Autodesk Fusion 360 part; units mm, degrees
sketch "base" plane through (0, 0, 0) normal (0, 0, 1) x (1, 0, 0)
  circle A0 centre (0, 0) radius 48
  circle A1 centre (0, 0) radius 37.5
  line L0 (0, 0) -> (0, 48)
  line L1 (0, 0) -> (-21.7169, 42.8063)
  line L2 (0, 0) -> (21.7169, 42.8063)
  dimension "d1" = 96
  dimension "d2" = 75
  dimension "d3" = 26.9
extrude "Extrude1" add sketch "base" against normal blind 15.5 contours A0 A1 L1 L2
extrude "Extrude2" add sketch "base" against normal blind 3 contours A1 L0 L2 | A1 L1 L2 | A1 L0 L1
sketch "axis" plane through (0, 0, 0) normal (0, 0, 1) x (1, 0, 0)
  circle A0 centre (0, 0) radius 10
  dimension "d8" = 20
extrude "Extrude3" add sketch "axis" along normal blind 20
fillet "Fillet1" radius 5 1 edges at (-9.3233, 3.6162, 0)
fillet "Fillet2" radius 1 1 edges at (-9.3233, -3.6162, 20)
sketch "thermal gaps" plane through (0, 0, 0) normal (0, 0, 1) x (1, 0, 0)
  line L0 (0, 0) -> (0, -65)
  line L1 (0, 0) -> (4.3074, -32.7177)
  line L2 (0, 0) -> (2.8716, -21.8118)
  line L3 (0, 0) -> (13.3928, -17.4538)
  line L4 (0, 0) -> (20.0891, -26.1807)
  arc A0 (2.8716, -21.8118) -> (13.3928, -17.4538) centre (0, 0) ccw
  arc A1 (4.3074, -32.7177) -> (20.0891, -26.1807) centre (0, 0) ccw
  line L5 (20.0891, -26.1807) -> (13.3928, -17.4538)
  line L6 (4.3074, -32.7177) -> (2.8716, -21.8118)
  line L7 (32.7177, -4.3074) -> (21.8118, -2.8716)
  line L8 (26.1807, -20.0891) -> (17.4538, -13.3928)
  arc A2 (17.4538, -13.3928) -> (21.8118, -2.8716) centre (0, 0) ccw
  arc A3 (26.1807, -20.0891) -> (32.7177, -4.3074) centre (0, 0) ccw
  line L9 (26.1807, 20.0891) -> (17.4538, 13.3928)
  line L10 (32.7177, 4.3074) -> (21.8118, 2.8716)
  arc A4 (21.8118, 2.8716) -> (17.4538, 13.3928) centre (0, 0) ccw
  arc A5 (32.7177, 4.3074) -> (26.1807, 20.0891) centre (0, 0) ccw
  line L11 (4.3074, 32.7177) -> (2.8716, 21.8118)
  line L12 (20.0891, 26.1807) -> (13.3928, 17.4538)
  arc A6 (13.3928, 17.4538) -> (2.8716, 21.8118) centre (0, 0) ccw
  arc A7 (20.0891, 26.1807) -> (4.3074, 32.7177) centre (0, 0) ccw
  line L13 (-20.0891, 26.1807) -> (-13.3928, 17.4538)
  line L14 (-4.3074, 32.7177) -> (-2.8716, 21.8118)
  arc A8 (-2.8716, 21.8118) -> (-13.3928, 17.4538) centre (0, 0) ccw
  arc A9 (-4.3074, 32.7177) -> (-20.0891, 26.1807) centre (0, 0) ccw
  line L15 (-32.7177, 4.3074) -> (-21.8118, 2.8716)
  line L16 (-26.1807, 20.0891) -> (-17.4538, 13.3928)
  arc A10 (-17.4538, 13.3928) -> (-21.8118, 2.8716) centre (0, 0) ccw
  arc A11 (-26.1807, 20.0891) -> (-32.7177, 4.3074) centre (0, 0) ccw
  line L17 (-26.1807, -20.0891) -> (-17.4538, -13.3928)
  line L18 (-32.7177, -4.3074) -> (-21.8118, -2.8716)
  arc A12 (-21.8118, -2.8716) -> (-17.4538, -13.3928) centre (0, 0) ccw
  arc A13 (-32.7177, -4.3074) -> (-26.1807, -20.0891) centre (0, 0) ccw
  line L19 (-4.3074, -32.7177) -> (-2.8716, -21.8118)
  line L20 (-20.0891, -26.1807) -> (-13.3928, -17.4538)
  arc A14 (-13.3928, -17.4538) -> (-2.8716, -21.8118) centre (0, 0) ccw
  arc A15 (-20.0891, -26.1807) -> (-4.3074, -32.7177) centre (0, 0) ccw
  dimension "d15" = 33
  dimension "d16" = 7.5
  dimension "d17" = 22
  dimension "d18" = 22
  dimension "d19" = 33
  dimension "d20" = 30
  dimension "d22" = 360
extrude "Extrude4" cut sketch "thermal gaps" against normal blind 10 contours L1 L4 A0 A1 L5 L6 | L7 L8 A2 A3 | L9 L10 A4 A5 | L11 L12 A6 A7 | L13 L14 A8 A9 | L15 L16 A10 A11 | L17 L18 A12 A13 | L19 L20 A14 A15
sketch "Sketch5" plane through (0, 0, 0) normal (0, 0, 1) x (1, 0, 0)
  line L0 (0, 0) -> (0, 42)
  circle A0 centre (0, 42) radius 2
  circle A1 centre (-29.6985, 29.6985) radius 2
  circle A2 centre (-42, 0) radius 2
  circle A3 centre (-29.6985, -29.6985) radius 2
  circle A4 centre (0, -42) radius 2
  circle A5 centre (29.6985, -29.6985) radius 2
  circle A6 centre (42, 0) radius 2
  circle A7 centre (29.6985, 29.6985) radius 2
  dimension "d25" = 42
  dimension "d26" = 4
  dimension "d28" = 360
extrude "Extrude5" cut sketch "Sketch5" against normal blind 25 contours A1 | A2 | A3 | A4 | A5 | A6 | A7
equation "d3 = ( 53.8 / 2 ) * 1 deg"
Check sheet for the modelled part. Datum: model origin and axes. Units: mm. A direction names the side the tool comes from. Round coordinates to 2 decimals unless told otherwise and drop trailing zeros. Order: outer loops, then holes, each group sorted by start corner. A loop starts at its lowest first (then second) coordinate and runs counter-clockwise, first axis right, second up. Notation, with made-up numbers: (66, -23) - (72, -23) arc R23 cw to (72, -15) - close; hole circle Ø4 at (-9, 44.25). An arc over 180 degrees is marked (long way). Write item = value, one per line.
Q1. Section check A-A (y = 0). Record the boundary of the cut face in (x, z).
Computed:
outline = (-48, -15.5) - (-44, -15.5) - (-44, 0) - (-48, 0) - close; (-40, -15.5) - (-37.5, -15.5) - (-37.5, -3) - (37.5, -3) - (37.5, -15.5) - (40, -15.5) - (40, 0) - (15, 0) arc R5 cw to (10, 5) - (10, 19) arc R1 ccw to (9, 20) - (-9, 20) arc R1 ccw to (-10, 19) - (-10, 5) arc R5 cw to (-15, 0) - (-40, 0) - close; (44, -15.5) - (48, -15.5) - (48, 0) - (44, 0) - close
Q2. Section check B-B (x = 0). Record the boundary of the cut face in (y, z), and give its area (3 significant figures).
Computed:
outline = (-48, -15.5) - (-44, -15.5) - (-44, 0) - (-48, 0) - close; (-40, -15.5) - (-37.5, -15.5) - (-37.5, -3) - (37.5, -3) - (37.5, 0) - (15, 0) arc R5 cw to (10, 5) - (10, 19) arc R1 ccw to (9, 20) - (-9, 20) arc R1 ccw to (-10, 19) - (-10, 5) arc R5 cw to (-15, 0) - (-40, 0) - close
area = 736 mm^2
Q3. Tool access check on faces 4 (the face through (-30.534, -12.517, -1.479)), 5 (the face through (-2.17, 9.76, 11.9)), 6 (the face through (19.31, 38.06, -7.64)). Record the directions out of +Z, -Z, +X, -X, +Y, -Y that give a thin tool (end or side, any length) a straight path to the whole face; none if there is none.
Computed:
face_4 = +Z, -Z
face_5 = +Z
face_6 = +Z, -Z, +Y
Q4. Thickness scan on line 1 along Y through (x, z) = (0, -5); line 2 along X through (y, z) = (-1.5, -4); line 3 along Y through (x, z) = (8, -1). Record the ranges inside material, lowest first.
Computed:
line_1 = -48 to -44, -40 to -37.5
line_2 = -47.98 to -43.32, -40.68 to -37.47, 37.47 to 40.68, 43.32 to 47.98
line_3 = -47.33 to -32.02, -20.49 to 20.49, 32.02 to 36.64
Q5. Go/stop test with flat-tipped pins: pin 1 (10 mm diameter, centred on x = -12, y = 19, fed in from +Z); pin 2 (5 mm diameter, centred on x = -24, y = -26, fed in from -Z); pin 3 (10 mm diameter, centred on y = 31, z = -9, fed in from +X); pin 4 (10 mm diameter, centred on x = -11.5, y = 21, fed in from -Z). Record where each tip stops, or that it passes through.
Computed:
pin_1 = 0
pin_2 = -15.5
pin_3 = 40.35
pin_4 = -3
Q6. Section check D-D (z = -9.5). Record the boundary of the cut face in (x, y).
Computed:
outline = (-21.72, 42.81) arc R48 ccw (long way) to (21.72, 42.81) - (16.97, 33.44) arc R37.5 cw (long way) to (-16.97, 33.44) - close; hole circle Ø4 at (-42, 0); hole circle Ø4 at (-29.7, -29.7); hole circle Ø4 at (-29.7, 29.7); hole circle Ø4 at (0, -42); hole circle Ø4 at (29.7, -29.7); hole circle Ø4 at (29.7, 29.7); hole circle Ø4 at (42, 0)
Q7. Draft check along Y on faces 1 (the face through (0, 0, 20)), 2 (the face through (30.774, 31.385, -7.642)), 3 (the face through (0.2, 37.5, -1.5)). Enter one of: pulls with the +Y half, pulls with the -Y half, needs draft (parallel to the pull), parting line crosses it, or undercut.
Computed:
face_1 = needs draft
face_2 = undercut
face_3 = pulls with the +Y half
Q8. Section check C-C (y = -42). Record the boundary of the cut face in (x, z).
Computed:
outline = (-23.24, -15.5) - (-2, -15.5) - (-2, 0) - (-23.24, 0) - close; (2, -15.5) - (23.24, -15.5) - (23.24, 0) - (2, 0) - close
